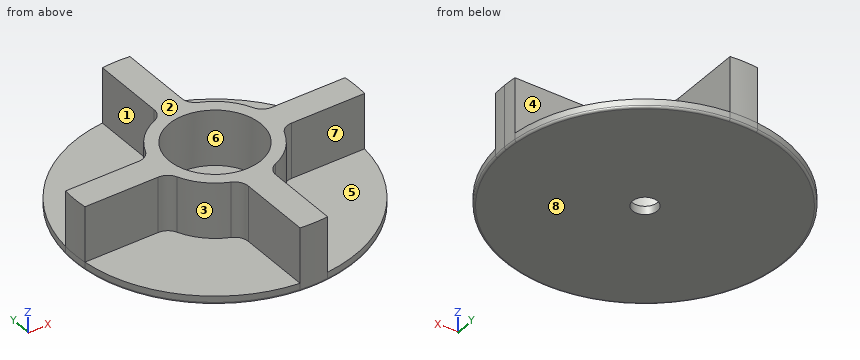
```python
from build123d import *

# Parameters (mm, degrees)
F0_R     = 6.65
F0_R_2   = 1.8
F1_DEPTH = 1.2
F2_DEPTH = 8
F3_R     = 0.3


# Not quite as in the source:
# - a feature names something its author has since deleted; it is built from what else it names


with BuildPart() as f1:
    # F0 (on Top) → F1 (new body)
    with BuildSketch(Plane.XY):
        with BuildLine():
            Line((9.6529388756, 1.998378199), (20.2717385681, 1.998378199))
            ThreePointArc((20.2717385681, 1.998378199), (14.4037651328, 14.4037651328), (1.998378199, 20.2717385681))
            Line((1.998378199, 20.2717385681), (1.998378199, 9.6529388756))
            ThreePointArc((1.998378199, 9.6529388756), (2.3354389744, 8.5417984096), (3.2330113343, 7.8051798106))
            ThreePointArc((3.2330113343, 7.8051798106), (5.9738260003, 5.9738260003), (7.8051798106, 3.2330113343))
            ThreePointArc((7.8051798106, 3.2330113343), (8.5417984096, 2.3354389744), (9.6529388756, 1.998378199))
        make_face()
        with BuildLine():
            Line((-1.998378199, 9.6529388756), (-1.998378199, 20.2717385681))
            ThreePointArc((-1.998378199, 20.2717385681), (-14.4037651328, 14.4037651328), (-20.2717385681, 1.998378199))
            Line((-20.2717385681, 1.998378199), (-9.6529388756, 1.998378199))
            ThreePointArc((-9.6529388756, 1.998378199), (-8.5417984096, 2.3354389744), (-7.8051798106, 3.2330113343))
            ThreePointArc((-7.8051798106, 3.2330113343), (-5.9738260003, 5.9738260003), (-3.2330113343, 7.8051798106))
            ThreePointArc((-3.2330113343, 7.8051798106), (-2.3354389744, 8.5417984096), (-1.998378199, 9.6529388756))
        make_face()
        with BuildLine():
            ThreePointArc((-20.2717385681, -1.998378199), (-14.4037651328, -14.4037651328), (-1.998378199, -20.2717385681))
            Line((-1.998378199, -20.2717385681), (-1.998378199, -9.6529388756))
            ThreePointArc((-1.998378199, -9.6529388756), (-2.3354389744, -8.5417984096), (-3.2330113343, -7.8051798106))
            ThreePointArc((-3.2330113343, -7.8051798106), (-5.9738260003, -5.9738260003), (-7.8051798106, -3.2330113343))
            ThreePointArc((-7.8051798106, -3.2330113343), (-8.5417984096, -2.3354389744), (-9.6529388756, -1.998378199))
            Line((-9.6529388756, -1.998378199), (-20.2717385681, -1.998378199))
        make_face()
        with BuildLine():
            ThreePointArc((1.998378199, -20.2717385681), (14.4037651328, -14.4037651328), (20.2717385681, -1.998378199))
            Line((20.2717385681, -1.998378199), (9.6529388756, -1.998378199))
            ThreePointArc((9.6529388756, -1.998378199), (8.5417984096, -2.3354389744), (7.8051798106, -3.2330113343))
            ThreePointArc((7.8051798106, -3.2330113343), (5.9738260003, -5.9738260003), (3.2330113343, -7.8051798106))
            ThreePointArc((3.2330113343, -7.8051798106), (2.3354389744, -8.5417984096), (1.998378199, -9.6529388756))
            Line((1.998378199, -9.6529388756), (1.998378199, -20.2717385681))
        make_face()
        with BuildLine():
            ThreePointArc((20.2717385681, -1.998378199), (20.3454198117, -1.0003962634), (20.37, 0))
            ThreePointArc((20.37, 0), (20.3454198117, 1.0003962634), (20.2717385681, 1.998378199))
            Line((20.2717385681, 1.998378199), (9.6529388756, 1.998378199))
            ThreePointArc((9.6529388756, 1.998378199), (8.5417984096, 2.3354389744), (7.8051798106, 3.2330113343))
            ThreePointArc((7.8051798106, 3.2330113343), (5.9738260003, 5.9738260003), (3.2330113343, 7.8051798106))
            ThreePointArc((3.2330113343, 7.8051798106), (2.3354389744, 8.5417984096), (1.998378199, 9.6529388756))
            Line((1.998378199, 9.6529388756), (1.998378199, 20.2717385681))
            ThreePointArc((1.998378199, 20.2717385681), (0, 20.37), (-1.998378199, 20.2717385681))
            Line((-1.998378199, 20.2717385681), (-1.998378199, 9.6529388756))
            ThreePointArc((-1.998378199, 9.6529388756), (-2.3354389744, 8.5417984096), (-3.2330113343, 7.8051798106))
            ThreePointArc((-3.2330113343, 7.8051798106), (-5.9738260003, 5.9738260003), (-7.8051798106, 3.2330113343))
            ThreePointArc((-7.8051798106, 3.2330113343), (-8.5417984096, 2.3354389744), (-9.6529388756, 1.998378199))
            Line((-9.6529388756, 1.998378199), (-20.2717385681, 1.998378199))
            ThreePointArc((-20.2717385681, 1.998378199), (-20.37, 0), (-20.2717385681, -1.998378199))
            Line((-20.2717385681, -1.998378199), (-9.6529388756, -1.998378199))
            ThreePointArc((-9.6529388756, -1.998378199), (-8.5417984096, -2.3354389744), (-7.8051798106, -3.2330113343))
            ThreePointArc((-7.8051798106, -3.2330113343), (-5.9738260003, -5.9738260003), (-3.2330113343, -7.8051798106))
            ThreePointArc((-3.2330113343, -7.8051798106), (-2.3354389744, -8.5417984096), (-1.998378199, -9.6529388756))
            Line((-1.998378199, -9.6529388756), (-1.998378199, -20.2717385681))
            ThreePointArc((-1.998378199, -20.2717385681), (0, -20.37), (1.998378199, -20.2717385681))
            Line((1.998378199, -20.2717385681), (1.998378199, -9.6529388756))
            ThreePointArc((1.998378199, -9.6529388756), (2.3354389744, -8.5417984096), (3.2330113343, -7.8051798106))
            ThreePointArc((3.2330113343, -7.8051798106), (5.9738260003, -5.9738260003), (7.8051798106, -3.2330113343))
            ThreePointArc((7.8051798106, -3.2330113343), (8.5417984096, -2.3354389744), (9.6529388756, -1.998378199))
            Line((9.6529388756, -1.998378199), (20.2717385681, -1.998378199))
        make_face()
        Circle(F0_R, mode=Mode.SUBTRACT)
        Circle(F0_R)
        Circle(F0_R_2, mode=Mode.SUBTRACT)
    extrude(amount=-F1_DEPTH)

    # F0 (on Top) → F2 (join)
    with BuildSketch(Plane.XY):
        with BuildLine():
            ThreePointArc((20.2717385681, -1.998378199), (20.3454198117, -1.0003962634), (20.37, 0))
            ThreePointArc((20.37, 0), (20.3454198117, 1.0003962634), (20.2717385681, 1.998378199))
            Line((20.2717385681, 1.998378199), (9.6529388756, 1.998378199))
            ThreePointArc((9.6529388756, 1.998378199), (8.5417984096, 2.3354389744), (7.8051798106, 3.2330113343))
            ThreePointArc((7.8051798106, 3.2330113343), (5.9738260003, 5.9738260003), (3.2330113343, 7.8051798106))
            ThreePointArc((3.2330113343, 7.8051798106), (2.3354389744, 8.5417984096), (1.998378199, 9.6529388756))
            Line((1.998378199, 9.6529388756), (1.998378199, 20.2717385681))
            ThreePointArc((1.998378199, 20.2717385681), (0, 20.37), (-1.998378199, 20.2717385681))
            Line((-1.998378199, 20.2717385681), (-1.998378199, 9.6529388756))
            ThreePointArc((-1.998378199, 9.6529388756), (-2.3354389744, 8.5417984096), (-3.2330113343, 7.8051798106))
            ThreePointArc((-3.2330113343, 7.8051798106), (-5.9738260003, 5.9738260003), (-7.8051798106, 3.2330113343))
            ThreePointArc((-7.8051798106, 3.2330113343), (-8.5417984096, 2.3354389744), (-9.6529388756, 1.998378199))
            Line((-9.6529388756, 1.998378199), (-20.2717385681, 1.998378199))
            ThreePointArc((-20.2717385681, 1.998378199), (-20.37, 0), (-20.2717385681, -1.998378199))
            Line((-20.2717385681, -1.998378199), (-9.6529388756, -1.998378199))
            ThreePointArc((-9.6529388756, -1.998378199), (-8.5417984096, -2.3354389744), (-7.8051798106, -3.2330113343))
            ThreePointArc((-7.8051798106, -3.2330113343), (-5.9738260003, -5.9738260003), (-3.2330113343, -7.8051798106))
            ThreePointArc((-3.2330113343, -7.8051798106), (-2.3354389744, -8.5417984096), (-1.998378199, -9.6529388756))
            Line((-1.998378199, -9.6529388756), (-1.998378199, -20.2717385681))
            ThreePointArc((-1.998378199, -20.2717385681), (0, -20.37), (1.998378199, -20.2717385681))
            Line((1.998378199, -20.2717385681), (1.998378199, -9.6529388756))
            ThreePointArc((1.998378199, -9.6529388756), (2.3354389744, -8.5417984096), (3.2330113343, -7.8051798106))
            ThreePointArc((3.2330113343, -7.8051798106), (5.9738260003, -5.9738260003), (7.8051798106, -3.2330113343))
            ThreePointArc((7.8051798106, -3.2330113343), (8.5417984096, -2.3354389744), (9.6529388756, -1.998378199))
            Line((9.6529388756, -1.998378199), (20.2717385681, -1.998378199))
        make_face()
        Circle(F0_R, mode=Mode.SUBTRACT)
    extrude(amount=F2_DEPTH)

    # F3
    f3_edges = [f1.edges().sort_by_distance(p)[0] for p in [
        (-1.998378, -20.271739, -1.2),
    ]]
    fillet(f3_edges, radius=F3_R)


solid = f1.part
```
For this review, take the finished solid that the model builds, in its own axes (mm). Face numbers are marked on the shaded views. A direction names the side the tool comes from. Give positions to 0.01 mm unless a question says otherwise; leave off trailing zeros. Write each loop counter-clockwise with the first axis right and the second up, starting at its lowest first coordinate (ties: lowest second). Pieces come first, ordered by that corner, then holes.
Item 1: Take a section at A-A (x = 0). Give the boundary of the cut face in (y, z).
Item 2: Insertion check: P1, Ø4, axis at y = 15, z = 5, coming from the +X side; P2, Ø2.5, axis at y = 17, z = 4, coming from the -X side; P3, Ø5.5, axis at x = 14.5, y = 8.5, coming from the +Z side. Each pin has a flat end and moves straight along its axis. Give the tip position at first contact, or say it passes through.
Item 3: Take a section at B-B (z = 4.25). Give the boundary of the cut face in (x, y), and give its area (3 significant figures).
Item 4: Wall thickness on probe 1 along Y at (x, z) = (0, 7.25); probe 2 along Y at (x, z) = (0, -0.3); probe 3 along Y at (x, z) = (13.5, 7.25): over which ranges is each line inside the solid? List them lowest first.
Item 5: The part is to be moulded in two halves that separate along Y. For the marked faces 6, 7 and 8, say which applies: +Y half, -Y half, draft (parallel to the pull), parting line (faces both ways), or undercut.
Item 6: Machinability: for the marked faces 1, 2, 3, 4 and 5, which of the approach directions +Z, -Z, +X, -X, +Y, -Y give a long, thin tool a straight path to every point of the face, cutting with its end or side? Answer none if there is none.
Established:
1. outline: (-20.37, -0.9) arc R0.3 ccw to (-20.07, -1.2) - (-1.8, -1.2) - (-1.8, 0) - (-6.65, 0) - (-6.65, 8) - (-20.37, 8) - close; (1.8, -1.2) - (20.07, -1.2) arc R0.3 ccw to (20.37, -0.9) - (20.37, 8) - (6.65, 8) - (6.65, 0) - (1.8, 0) - close
2. P1: stops at x = 2
2. P2: stops at x = -2
2. P3: stops at z = 0
3. outline: (-20.27, -2) - (-9.65, -2) arc R2 cw to (-7.81, -3.23) arc R8.45 ccw to (-3.23, -7.81) arc R2 cw to (-2, -9.65) - (-2, -20.27) arc R20.37 ccw to (2, -20.27) - (2, -9.65) arc R2 cw to (3.23, -7.81) arc R8.45 ccw to (7.81, -3.23) arc R2 cw to (9.65, -2) - (20.27, -2) arc R20.37 ccw to (20.27, 2) - (9.65, 2) arc R2 cw to (7.81, 3.23) arc R8.45 ccw to (3.23, 7.81) arc R2 cw to (2, 9.65) - (2, 20.27) arc R20.37 ccw to (-2, 20.27) - (-2, 9.65) arc R2 cw to (-3.23, 7.81) arc R8.45 ccw to (-7.81, 3.23) arc R2 cw to (-9.65, 2) - (-20.27, 2) arc R20.37 ccw to start; hole circle Ø13.3 at (0, 0)
3. area: 280 mm2
4. probe 1: y = -20.37 to -6.65, 6.65 to 20.37
4. probe 2: y = -20.37 to -1.8, 1.8 to 20.37
4. probe 3: y = -2 to 2
5. face 6: undercut
5. face 7: -Y half
5. face 8: draft
6. face 1: +Z, -X, +Y
6. face 2: +Z, +X, -X, +Y, -Y
6. face 3: +Z, -X, -Y
6. face 4: +Z, +X, +Y
6. face 5: +Z, +X, -Y
